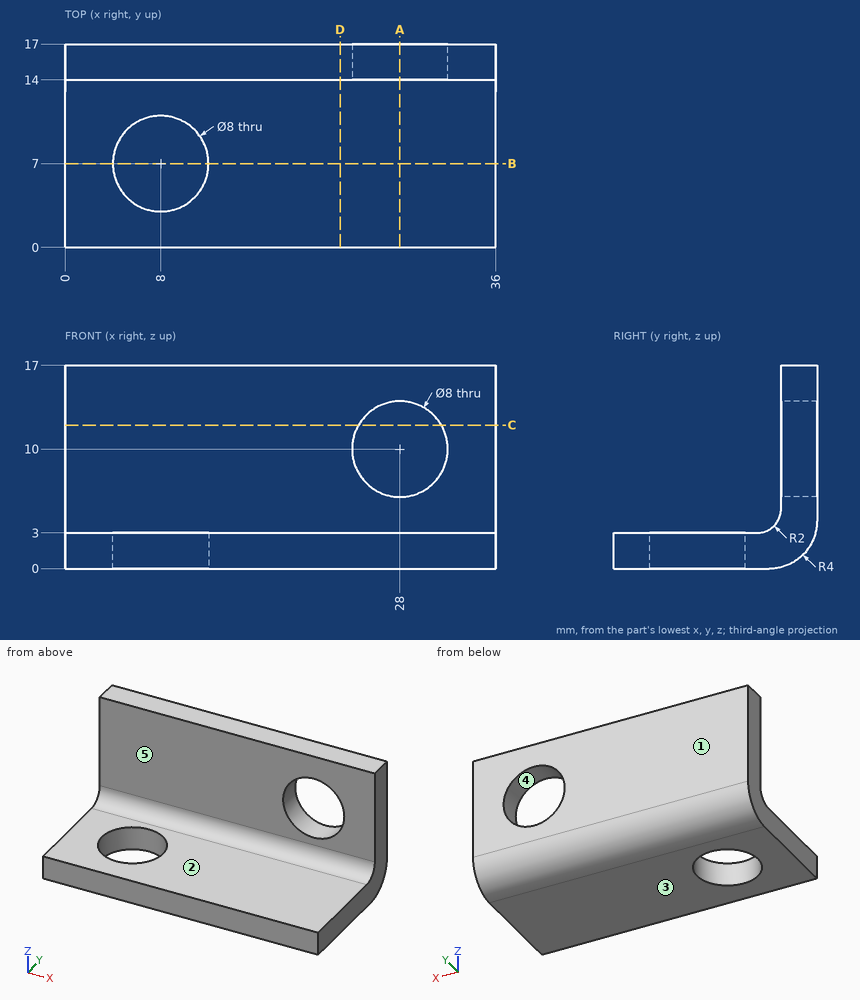
Answer from the drawing. Dimensions are ordinates in mm from the lowest x, y and z of the part. A direction names the side the tool comes from. Give positions to 0.01 mm unless a question says otherwise; leave off trailing zeros. Order: outer loops, then holes, each group sorted by start corner. A loop starts at its lowest first (then second) coordinate and runs counter-clockwise, first axis right, second up. Notation, with made-up numbers: (71.5, -28.75) -> (95.5, -28.75) arc R16 cw to (95.5, -10.75) -> close; hole circle Ø4 at (50.25, -21.5). An arc over 180 degrees is marked (long way). One line per item, written item: value. Start each with the question number.
(1) The part is cut by section B-B (y = 7). Determine the outline of the cut face in (x, z).
(2) The part is cut by section C-C (z = 12). Determine the outline of the cut face in (x, y), and give its area (3 significant figures).
(3) Straight lines are drawn through the part: L1, parallel to Z at x = 7.5, y = 1.75; L2, parallel to Y at x = 18, z = 11.25; L3, parallel to Z at x = 28, y = 16.15. For each, find the intervals that lie inside material, in ascending order.
(4) For a pull along Z with two mould halves and no side action, classify the marked faces 3, 4 and 5 as released by +Z, released by -Z, zero draft, split by the parting line, or undercut.
(5) The part is cut by section A-A (x = 28). Determine the outline of the cut face in (y, z).
(6) The part is cut by section D-D (x = 23). Determine the outline of the cut face in (y, z), and give its area (3 significant figures).
(7) Flat-ended cylindrical pins translate along their axes: P1, Ø7, axis at x = 28, z = 10, coming from the +Y side (3 decimals); P2, Ø2, axis at x = 4.5, z = 4.5, coming from the -Y side; P3, Ø6, axis at x = 10.5, y = 6, coming from the +Z side. Find the tip coordinate at first contact, or state that the pin passes through.
(8) A tool of negligible diameter and unlimited length cuts with its end or side. For the marked faces 1 and 2, from which of +Z, -Z, +X, -X, +Y, -Y can it reach the whole face along a straight path? Write none if from no direction.
Taken from the geometry:
1. outline: (0, 0) -> (4, 0) -> (4, 3) -> (0, 3) -> close; (12, 0) -> (36, 0) -> (36, 3) -> (12, 3) -> close
2. outline: (0, 14) -> (24.54, 14) -> (24.54, 17) -> (0, 17) -> close; (31.46, 14) -> (36, 14) -> (36, 17) -> (31.46, 17) -> close
2. area: 87.2 mm^2
3. L1: 0 to 3
3. L2: 14 to 17
3. L3: 1.53 to 6, 14 to 17
4. face 3: released by -Z
4. face 4: undercut
4. face 5: zero draft
5. outline: (0, 0) -> (13, 0) arc R4 ccw to (17, 4) -> (17, 6) -> (14, 6) -> (14, 5) arc R2 cw to (12, 3) -> (0, 3) -> close; (14, 14) -> (17, 14) -> (17, 17) -> (14, 17) -> close
6. outline: (0, 0) -> (13, 0) arc R4 ccw to (17, 4) -> (17, 17) -> (14, 17) -> (14, 5) arc R2 cw to (12, 3) -> (0, 3) -> close
6. area: 90.4 mm^2
7. P1: through
7. P2: y = 13.32
7. P3: z = 3
8. face 1: +Z, -Z, +X, -X, +Y
8. face 2: +Z, +X, -X, -Y
